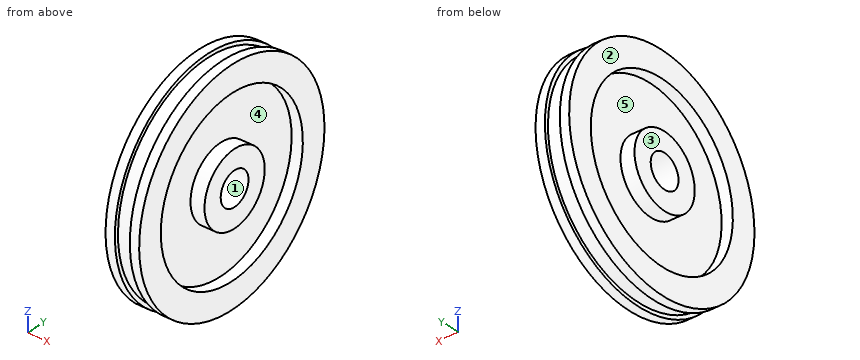
from build123d import *


with BuildPart() as part:
    # Esquisse1 → Révolution1 (revolve)
    with BuildSketch(Plane.XY, mode=Mode.PRIVATE) as r_volution1_sk:
        Polygon((0, 0), (21, 0), (21, 10.5), (13.5, 10.5), (13.5, 37), (19.5, 37), (19.5, 51), (14.5, 51), (14.5, 49), (6.5, 49), (6.5, 51), (1.5, 51), (1.5, 37), (7.5, 37), (7.5, 10.5), (0, 10.5), align=None)
    revolve(r_volution1_sk.sketch.rotate(Axis((0, -9, 0), (1, 0, 0)), 90), axis=Axis((0, -9, 0), (1, 0, 0)))


solid = part.part
Can you work these out from the model? Positions are in its coordinate system, mm. Face numbers are marked on the shaded views. A direction names the side the tool comes from. Coordinates: 2 decimals unless noted, no trailing zeros. Order: outer loops, then holes, each group sorted by start corner. A loop starts at its lowest first (then second) coordinate and runs counter-clockwise, first axis right, second up. Notation, with made-up numbers: (-10, 78.25) - (11, 78.25) arc R26 cw to (11, 105.25) - close; hole circle Ø10 at (13.5, 73.25). An arc over 180 degrees is marked (long way). Answer as a JSON object with one key per item and string values. Group by question number.
Q1. Imagine slicing it at D-D (y = 33.5). Please give me the cut outline in (x, z), and give its area (3 significant figures).
Q2. Imagine slicing it at C-C (x = 16). Please give me the cut outline in (y, z), and give its area (3 significant figures).
Q3. I need wall thicknesses on line 1 (Y direction, x = 5.7, z = 0); line 2 (X direction, y = -58, z = -6.5); line 3 (Y direction, x = 3.25, z = 10). Which ranges of each line are inside material? Lowest first, please. Write a range as from..to.
Q4. On a 3-axis mill with a long thin cutter (end or side, diameter ignored), from which of +Z, -Z, +X, -X, +Y, -Y can I reach the whole of each face in a straight line? I mean the marked faces 3, 4 and 5. Say none if no direction works.
Q5. Will these pins go through, and if not, where does the flat tip stop? P1, Ø3, axis at y = 21, z = -25.5, coming from the +X side; P2, Ø10, axis at x = 7, y = 5, coming from the -Z side; P3, Ø4, axis at x = 14.5, y = 23, coming from the +Z side; P4, Ø11, axis at y = -9, z = 0, coming from the +X side.
Q6. We'd pull the mould along Z, two halves only. Please class the marked faces 1 and 2: +Z half, -Z half, draft (parallel to the pull), parting line (faces both ways), or undercut.
Determined:
{
 "1": {"outline": "(1.5, -42.35) - (6.5, -42.35) - (6.5, -39.47) - (14.5, -39.47) - (14.5, -42.35) - (19.5, -42.35) - (19.5, -17.6) - (13.5, -17.6) - (13.5, 17.6) - (19.5, 17.6) - (19.5, 42.35) - (14.5, 42.35) - (14.5, 39.47) - (6.5, 39.47) - (6.5, 42.35) - (1.5, 42.35) - (1.5, 17.6) - (7.5, 17.6) - (7.5, -17.6) - (1.5, -17.6) - close", "area": "1,060 mm2"},
 "2": {"outline": "circle Ø120 at (-9, 0); circle Ø39 at (-9, 0); hole circle Ø92 at (-9, 0); hole circle Ø18 at (-9, 0)", "area": "5,600 mm2"},
 "3": {"line 1": "y = -69..-55, -28.5..-18, 0..10.5, 37..51", "line 2": "x = 1.5..19.5", "line 3": "y = -68.16..-53.9, -25.74..7.74, 35.9..50.16"},
 "4": {"face 3": "+Z, -Z, -X, +Y, -Y", "face 4": "+X", "face 5": "-X"},
 "5": {"P1": "stops at x = 13.5", "P2": "stops at z = -59.32", "P3": "stops at z = 51.96", "P4": "passes through"},
 "6": {"face 1": "undercut", "face 2": "draft"}
}
